Read the model definition and answer for the solid it produces. Units are mm, in the model's axes. Coordinates: 2 decimals unless noted, no trailing zeros.
Autodesk Inventor part; units mm, degrees
ref_plane "YZ Plane" through (0, 0, 0) normal (1, 0, 0) x (0, 1, 0)
ref_plane "XZ Plane" through (0, 0, 0) normal (0, 1, 0) x (-1, 0, 0)
ref_plane "XY Plane" through (0, 0, 0) normal (0, 0, 1) x (1, 0, 0)
sketch "T-Slot 4040 Base" plane through (0, 0, 0) normal (0, 0, 1) x (1, 0, 0)
  line L0 (-28, 0) -> (28, 0) construction
  line L1 (0, -28) -> (0, 28) construction
  circle A0 centre (0, 0) radius 5.1
  line L2 (-7.5, -7.5) -> (7.5, -7.5)
  line L3 (7.5, -7.5) -> (7.5, 7.5)
  line L4 (7.5, 7.5) -> (-7.5, 7.5)
  line L5 (-7.5, 7.5) -> (-7.5, -7.5)
  line L6 (-7.5, -7.5) -> (7.5, 7.5) construction
  line L7 (7.5, -7.5) -> (-7.5, 7.5) construction
  line L8 (-20, 20) -> (20, 20)
  line L9 (20, 20) -> (20, -20)
  line L10 (20, -20) -> (-20, -20)
  line L11 (-20, -20) -> (-20, 20)
  line L12 (-20, 20) -> (20, -20) construction
  line L13 (20, 20) -> (-20, -20) construction
  line L14 (20, 5) -> (14.5, 5)
  line L15 (14.5, 5) -> (14.5, 10)
  line L16 (14.5, 10) -> (12.4749, 10)
  line L17 (12.4749, 10) -> (7.5, 5.0251)
  line L18 (5, 20) -> (5, 14.5)
  line L19 (5, 14.5) -> (10, 14.5)
  line L20 (10, 14.5) -> (10, 12.4749)
  line L21 (10, 12.4749) -> (5.0251, 7.5)
  line L22 (18.5, 18.5) -> (11.5, 18.5)
  line L23 (11.5, 18.5) -> (11.5, 11.5)
  line L24 (11.5, 11.5) -> (18.5, 11.5)
  line L25 (18.5, 11.5) -> (18.5, 18.5)
  line L26 (18.5, 18.5) -> (11.5, 11.5) construction
  line L27 (11.5, 18.5) -> (18.5, 11.5) construction
  line L28 (3.0732, 1.3088) -> (4.38, 2.6125) construction
  line L29 (5.905, 4.1338) -> (4.1393, 5.9037)
  line L30 (4.1393, 5.9037) -> (2.6122, 4.3802)
  line L31 (1.3075, 3.0787) -> (3.0732, 1.3088) construction
  line L32 (3.0732, 1.3088) -> (4.1393, 5.9037) construction
  line L33 (5.905, 4.1338) -> (1.3075, 3.0787) construction
  line L34 (4.38, 2.6125) -> (5.905, 4.1338)
  line L35 (2.6122, 4.3802) -> (1.3075, 3.0787) construction
  line L36 (-20, 5) -> (-14.5, 5)
  line L37 (-14.5, 5) -> (-14.5, 10)
  line L38 (-14.5, 10) -> (-12.4749, 10)
  line L39 (-12.4749, 10) -> (-7.5, 5.0251)
  line L40 (-5, 20) -> (-5, 14.5)
  line L41 (-5, 14.5) -> (-10, 14.5)
  line L42 (-10, 14.5) -> (-10, 12.4749)
  line L43 (-10, 12.4749) -> (-5.0251, 7.5)
  line L44 (-18.5, 18.5) -> (-11.5, 18.5)
  line L45 (-11.5, 18.5) -> (-11.5, 11.5)
  line L46 (-11.5, 11.5) -> (-18.5, 11.5)
  line L47 (-18.5, 11.5) -> (-18.5, 18.5)
  line L48 (-5.905, 4.1338) -> (-4.1393, 5.9037)
  line L49 (-4.1393, 5.9037) -> (-2.6122, 4.3802)
  line L50 (-4.38, 2.6125) -> (-5.905, 4.1338)
  line L51 (7.5, -7.5) -> (-7.5, -7.5)
  line L52 (20, -5) -> (14.5, -5)
  line L53 (14.5, -5) -> (14.5, -10)
  line L54 (14.5, -10) -> (12.4749, -10)
  line L55 (12.4749, -10) -> (7.5, -5.0251)
  line L56 (5, -20) -> (5, -14.5)
  line L57 (5, -14.5) -> (10, -14.5)
  line L58 (10, -14.5) -> (10, -12.4749)
  line L59 (10, -12.4749) -> (5.0251, -7.5)
  line L60 (18.5, -18.5) -> (11.5, -18.5)
  line L61 (11.5, -18.5) -> (11.5, -11.5)
  line L62 (11.5, -11.5) -> (18.5, -11.5)
  line L63 (18.5, -11.5) -> (18.5, -18.5)
  line L64 (18.5, -18.5) -> (11.5, -11.5) construction
  line L65 (11.5, -18.5) -> (18.5, -11.5) construction
  line L66 (3.0732, -1.3088) -> (4.38, -2.6125) construction
  line L67 (5.905, -4.1338) -> (4.1393, -5.9037)
  line L68 (4.1393, -5.9037) -> (2.6122, -4.3802)
  line L69 (1.3075, -3.0787) -> (3.0732, -1.3088) construction
  line L70 (3.0732, -1.3088) -> (4.1393, -5.9037) construction
  line L71 (5.905, -4.1338) -> (1.3075, -3.0787) construction
  line L72 (4.38, -2.6125) -> (5.905, -4.1338)
  line L73 (2.6122, -4.3802) -> (1.3075, -3.0787) construction
  line L74 (-4.38, -2.6125) -> (-5.905, -4.1338)
  line L75 (-4.1393, -5.9037) -> (-2.6122, -4.3802)
  line L76 (-5.905, -4.1338) -> (-4.1393, -5.9037)
  line L77 (-12.4749, -10) -> (-7.5, -5.0251)
  line L78 (-10, -12.4749) -> (-5.0251, -7.5)
  line L79 (-10, -14.5) -> (-10, -12.4749)
  line L80 (-5, -14.5) -> (-10, -14.5)
  line L81 (-5, -20) -> (-5, -14.5)
  line L82 (-18.5, -18.5) -> (-11.5, -18.5)
  line L83 (-11.5, -18.5) -> (-11.5, -11.5)
  line L84 (-11.5, -11.5) -> (-18.5, -11.5)
  line L85 (-18.5, -11.5) -> (-18.5, -18.5)
  line L86 (-14.5, -10) -> (-12.4749, -10)
  line L87 (-14.5, -5) -> (-14.5, -10)
  line L88 (-20, -5) -> (-14.5, -5)
  point P0 (15, 15)
  point P1 (3.6062, 3.6062)
  point P2 (3.6062, 3.6062)
  point P3 (15, -15)
  point P4 (3.6062, -3.6062)
  point P5 (3.6062, -3.6062)
  dimension "d9" = 10.2
  dimension "d12" = 40
  dimension "d13" = 40
  dimension "d14" = 5.5
  dimension "d15" = 15
  dimension "d16" = 7
  dimension "d17" = 10
  dimension "d20" = 1.75
  dimension "d21" = 7
  dimension "d22" = 2
  dimension "d29" = 1.5
  dimension "d30" = 2.5
extrude "Extrusion1" add sketch "T-Slot 4040 Base" along normal blind 1357 contours L5 L4 L3 L2 | L2 L78 L79 L80 L81 L10 L11 L88 L87 L86 L77 L5 | L2 L3 L55 L54 L53 L52 L9 L10 L56 L57 L58 L59 | L39 L38 L37 L36 L11 L8 L40 L41 L42 L43 L4 L5 | L3 L4 L21 L20 L19 L18 L8 L9 L14 L15 L16 L17
fillet "Rundung1" radius 1 16 edges at (11.5, 18.5, 678.5) (18.5, 18.5, 678.5) (18.5, 11.5, 678.5) (11.5, 11.5, 678.5) (-11.5, 18.5, 678.5) (-18.5, 18.5, 678.5) (-18.5, 11.5, 678.5) (-11.5, 11.5, 678.5) (-18.5, -11.5, 678.5) (-11.5, -11.5, 678.5) (-11.5, -18.5, 678.5) (-18.5, -18.5, 678.5) (11.5, -18.5, 678.5) (11.5, -11.5, 678.5) (18.5, -11.5, 678.5) (18.5, -18.5, 678.5)
fillet "Rundung2" radius 3 4 edges at (20, 20, 678.5) (20, -20, 678.5) (-20, -20, 678.5) (-20, 20, 678.5)
properties part number "T-SLOT 4040 B-Type 1357mm"
Item 1: Given pin 1 (3 mm diameter, centred on x = 2, z = 926.5, fed in from -Y); pin 2 (6 mm diameter, centred on y = -0.5, z = 798, fed in from +X); pin 3 (4 mm diameter, centred on y = -1.5, z = 832, fed in from -X), each flat-ended and moving along its own axis, determine where each tip first touches the part or whether it passes through.
Numbers:
pin 1: stops at y = -7.5
pin 2: stops at x = 7.5
pin 3: stops at x = -7.5
Item 2: A cutting plane is placed at A-A on z = 854.5. Give the number of separate pieces and of enclosed holes in the cut face, then the cut area to 3 significant figures.
Numbers:
separate pieces: 1
enclosed holes: 5
area: 616 mm2
Item 3: Find the intervals of material crossed by line 1 along X through (y, z) = (-12.5, 813.5); line 2 along Y through (x, z) = (-18, 335); line 3 along X through (y, z) = (16.5, 489), in increasing order.
Numbers:
line 1: x = -20 to -18.5, -11.5 to -10, 10 to 11.5, 18.5 to 20
line 2: y = -19.83 to -18.37, -11.63 to -5, 5 to 11.63, 18.37 to 19.83
line 3: x = -20 to -18.5, -11.5 to -5, 5 to 11.5, 18.5 to 20
